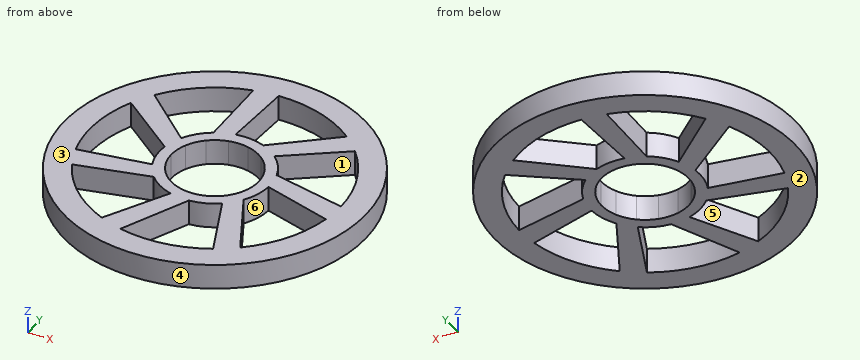
```python
from build123d import *

# Parameters (mm, degrees)
F0_R     = 38.1
F1_DEPTH = 6.35


with BuildPart() as f1:
    # F0 (on Top) → F1 (new body)
    with BuildSketch(Plane.XY):
        Circle(F0_R)
        with BuildLine():
            ThreePointArc((31.7250303997, 0), (31.5812646245, -3.0168325409), (31.1512702825, -6.0063228058))
            ThreePointArc((31.1512702825, -6.0063228058), (27.1447816525, -16.4206693804), (19.7802329179, -24.8036275488))
            ThreePointArc((19.7802329179, -24.8036275488), (17.3319417654, -26.5721912628), (14.7265670727, -28.0999248419))
            ThreePointArc((14.7265670727, -28.0999248419), (4.0862982493, -31.460764779), (-7.0594833943, -30.9296176515))
            ThreePointArc((-7.0594833943, -30.9296176515), (-9.9686867503, -30.1181479898), (-12.7875415101, -29.033710338))
            ThreePointArc((-12.7875415101, -29.033710338), (-22.049251081, -22.8102626164), (-28.5832647234, -13.7649748135))
            ThreePointArc((-28.5832647234, -13.7649748135), (-29.7626908188, -10.9845249823), (-30.6723705175, -8.1045197699))
            ThreePointArc((-30.6723705175, -8.1045197699), (-31.5812646245, 3.0168325409), (-28.5832647234, 13.7649748135))
            ThreePointArc((-28.5832647234, 13.7649748135), (-27.1447816525, 16.4206693804), (-25.4602789229, 18.9275394871))
            ThreePointArc((-25.4602789229, 18.9275394871), (-17.3319417654, 26.5721912628), (-7.0594833943, 30.9296176515))
            ThreePointArc((-7.0594833943, 30.9296176515), (-4.0862982493, 31.460764779), (-1.0760780042, 31.7067754588))
            ThreePointArc((-1.0760780042, 31.7067754588), (9.9686867503, 30.1181479898), (19.7802329179, 24.8036275488))
            ThreePointArc((19.7802329179, 24.8036275488), (22.049251081, 22.8102626164), (24.1184315996, 20.6101628097))
            ThreePointArc((24.1184315996, 20.6101628097), (29.7626908188, 10.9845249823), (31.7250303997, 0))
        make_face(mode=Mode.SUBTRACT)
        with BuildLine():
            Line((-10.2881439148, -9.4506610768), (-6.878658835, -8.6466440676))
            ThreePointArc((-6.878658835, -8.6466440676), (-8.634357457, -6.8940751595), (-9.9548050215, -4.7939814335))
            Line((-9.9548050215, -4.7939814335), (-12.9376014162, -5.270613778))
            ThreePointArc((-12.9376014162, -5.270613778), (-11.7994495804, -7.4788962822), (-10.2881439148, -9.4506610768))
        make_face()
        with BuildLine():
            Line((-28.5832647234, -13.7649748135), (-10.2881439148, -9.4506610768))
            ThreePointArc((-10.2881439148, -9.4506610768), (-11.7994495804, -7.4788962822), (-12.9376014162, -5.270613778))
            Line((-12.9376014162, -5.270613778), (-30.6723705175, -8.1045197699))
            ThreePointArc((-30.6723705175, -8.1045197699), (-29.7626908188, -10.9845249823), (-28.5832647234, -13.7649748135))
        make_face()
        with BuildLine():
            ThreePointArc((-11.0489921838, -0.0131423621), (-10.7734388222, 2.4522269355), (-9.9548050215, 4.7939814335))
            Line((-9.9548050215, 4.7939814335), (-12.187194327, 6.8288501547))
            ThreePointArc((-12.187194327, 6.8288501547), (-13.2040730485, 4.5621655966), (-13.8033771709, 2.1512040066))
            Line((-13.8033771709, 2.1512040066), (-11.0489921838, -0.0131423621))
        make_face()
        with BuildLine():
            ThreePointArc((-13.8033771709, 2.1512040066), (-13.2040730485, 4.5621655966), (-12.187194327, 6.8288501547))
            Line((-12.187194327, 6.8288501547), (-25.4602789229, 18.9275394871))
            ThreePointArc((-25.4602789229, 18.9275394871), (-27.1447816525, 16.4206693804), (-28.5832647234, 13.7649748135))
            Line((-28.5832647234, 13.7649748135), (-13.8033771709, 2.1512040066))
        make_face()
        with BuildLine():
            ThreePointArc((-6.8992090599, 8.6302558101), (-4.7999010163, 9.9519521318), (-2.4586337993, 10.7719785017))
            Line((-2.4586337993, 10.7719785017), (-2.2595813362, 13.7860506377))
            ThreePointArc((-2.2595813362, 13.7860506377), (-4.665760197, 13.16782373), (-6.9243858797, 12.1331685964))
            Line((-6.9243858797, 12.1331685964), (-6.8992090599, 8.6302558101))
        make_face()
        with BuildLine():
            ThreePointArc((-6.9243858797, 12.1331685964), (-4.665760197, 13.16782373), (-2.2595813362, 13.7860506377))
            Line((-2.2595813362, 13.7860506377), (-1.0760780042, 31.7067754588))
            ThreePointArc((-1.0760780042, 31.7067754588), (-4.0862982493, 31.460764779), (-7.0594833943, 30.9296176515))
            Line((-7.0594833943, 30.9296176515), (-6.9243858797, 12.1331685964))
        make_face()
        with BuildLine():
            ThreePointArc((2.4458192044, 10.7748953322), (4.7880601551, 9.95765439), (6.8889388207, 8.6384560498))
            Line((6.8889388207, 8.6384560498), (9.3695424879, 10.3620738064))
            ThreePointArc((9.3695424879, 10.3620738064), (7.3859652469, 11.85784202), (5.1688092106, 12.9786097616))
            Line((5.1688092106, 12.9786097616), (2.4458192044, 10.7748953322))
        make_face()
        with BuildLine():
            ThreePointArc((5.1688092106, 12.9786097616), (7.3859652469, 11.85784202), (9.3695424879, 10.3620738064))
            Line((9.3695424879, 10.3620738064), (24.1184315996, 20.6101628097))
            ThreePointArc((24.1184315996, 20.6101628097), (22.049251081, 22.8102626164), (19.7802329179, 24.8036275488))
            Line((19.7802329179, 24.8036275488), (5.1688092106, 12.9786097616))
        make_face()
        with BuildLine():
            ThreePointArc((9.9490957221, 4.8058189013), (10.770514371, 2.4650397934), (11.049, 0))
            Line((11.049, 0), (13.9432097147, -0.864755949))
            ThreePointArc((13.9432097147, -0.864755949), (13.9633008224, -0.4325854166), (13.97, 0))
            ThreePointArc((13.97, 0), (13.8191317384, 2.0475590338), (13.3697855409, 4.0508930609))
            Line((13.3697855409, 4.0508930609), (9.9490957221, 4.8058189013))
        make_face()
        with BuildLine():
            ThreePointArc((13.97, 0), (13.9633008224, -0.4325854166), (13.9432097147, -0.864755949))
            Line((13.9432097147, -0.864755949), (31.1512702825, -6.0063228058))
            ThreePointArc((31.1512702825, -6.0063228058), (31.5812646245, -3.0168325409), (31.7250303997, 0))
            Line((31.7250303997, 0), (13.3697855409, 4.0508930609))
            ThreePointArc((13.3697855409, 4.0508930609), (13.8191317384, 2.0475590338), (13.97, 0))
        make_face()
        with BuildLine():
            Line((11.5030406649, -7.9272287378), (9.9605002365, -4.7821371831))
            ThreePointArc((9.9605002365, -4.7821371831), (8.6425515871, -6.8838000453), (6.8889388207, -8.6384560498))
            Line((6.8889388207, -8.6384560498), (8.0173556368, -11.4404068369))
            ThreePointArc((8.0173556368, -11.4404068369), (9.9170092786, -9.8394017586), (11.5030406649, -7.9272287378))
        make_face()
        with BuildLine():
            Line((19.7802329179, -24.8036275488), (11.5030406649, -7.9272287378))
            ThreePointArc((11.5030406649, -7.9272287378), (9.9170092786, -9.8394017586), (8.0173556368, -11.4404068369))
            Line((8.0173556368, -11.4404068369), (14.7265670727, -28.0999248419))
            ThreePointArc((14.7265670727, -28.0999248419), (17.3319417654, -26.5721912628), (19.7802329179, -24.8036275488))
        make_face()
        with BuildLine():
            Line((0.974271549, -13.935985611), (2.4714449156, -10.7690464308))
            ThreePointArc((2.4714449156, -10.7690464308), (0.0065711822, -11.048998046), (-2.4586337993, -10.7719785017))
            Line((-2.4586337993, -10.7719785017), (-3.9457307599, -13.4011980349))
            ThreePointArc((-3.9457307599, -13.4011980349), (-1.5095999134, -13.8881967189), (0.974271549, -13.935985611))
        make_face()
        with BuildLine():
            Line((-7.0594833943, -30.9296176515), (0.974271549, -13.935985611))
            ThreePointArc((0.974271549, -13.935985611), (-1.5095999134, -13.8881967189), (-3.9457307599, -13.4011980349))
            Line((-3.9457307599, -13.4011980349), (-12.7875415101, -29.033710338))
            ThreePointArc((-12.7875415101, -29.033710338), (-9.9686867503, -30.1181479898), (-7.0594833943, -30.9296176515))
        make_face()
        with BuildLine():
            ThreePointArc((-9.9548050215, 4.7939814335), (-8.6425515871, 6.8838000453), (-6.8992090599, 8.6302558101))
            Line((-6.8992090599, 8.6302558101), (-6.9243858797, 12.1331685964))
            ThreePointArc((-6.9243858797, 12.1331685964), (-9.9170092786, 9.8394017586), (-12.187194327, 6.8288501547))
            Line((-12.187194327, 6.8288501547), (-9.9548050215, 4.7939814335))
        make_face()
        with BuildLine():
            Line((-12.9376014162, -5.270613778), (-9.9548050215, -4.7939814335))
            ThreePointArc((-9.9548050215, -4.7939814335), (-10.770514371, -2.4650397934), (-11.0489921838, -0.0131423621))
            Line((-11.0489921838, -0.0131423621), (-13.8033771709, 2.1512040066))
            ThreePointArc((-13.8033771709, 2.1512040066), (-13.8759082137, -1.6186634131), (-12.9376014162, -5.270613778))
        make_face()
        with BuildLine():
            Line((-3.9457307599, -13.4011980349), (-2.4586337993, -10.7719785017))
            ThreePointArc((-2.4586337993, -10.7719785017), (-4.7880601551, -9.95765439), (-6.878658835, -8.6466440676))
            Line((-6.878658835, -8.6466440676), (-10.2881439148, -9.4506610768))
            ThreePointArc((-10.2881439148, -9.4506610768), (-7.3859652469, -11.85784202), (-3.9457307599, -13.4011980349))
        make_face()
        with BuildLine():
            Line((8.0173556368, -11.4404068369), (6.8889388207, -8.6384560498))
            ThreePointArc((6.8889388207, -8.6384560498), (4.7999010163, -9.9519521318), (2.4714449156, -10.7690464308))
            Line((2.4714449156, -10.7690464308), (0.974271549, -13.935985611))
            ThreePointArc((0.974271549, -13.935985611), (4.665760197, -13.16782373), (8.0173556368, -11.4404068369))
        make_face()
        with BuildLine():
            Line((13.9432097147, -0.864755949), (11.049, 0))
            ThreePointArc((11.049, 0), (10.7734388222, -2.4522269355), (9.9605002365, -4.7821371831))
            Line((9.9605002365, -4.7821371831), (11.5030406649, -7.9272287378))
            ThreePointArc((11.5030406649, -7.9272287378), (13.2040730485, -4.5621655966), (13.9432097147, -0.864755949))
        make_face()
        with BuildLine():
            ThreePointArc((6.8889388207, 8.6384560498), (8.634357457, 6.8940751595), (9.9490957221, 4.8058189013))
            Line((9.9490957221, 4.8058189013), (13.3697855409, 4.0508930609))
            ThreePointArc((13.3697855409, 4.0508930609), (11.7994495804, 7.4788962822), (9.3695424879, 10.3620738064))
            Line((9.3695424879, 10.3620738064), (6.8889388207, 8.6384560498))
        make_face()
        with BuildLine():
            ThreePointArc((-2.4586337993, 10.7719785017), (-0.0065711822, 11.048998046), (2.4458192044, 10.7748953322))
            Line((2.4458192044, 10.7748953322), (5.1688092106, 12.9786097616))
            ThreePointArc((5.1688092106, 12.9786097616), (1.5095999134, 13.8881967189), (-2.2595813362, 13.7860506377))
            Line((-2.2595813362, 13.7860506377), (-2.4586337993, 10.7719785017))
        make_face()
    extrude(amount=F1_DEPTH)


solid = f1.part
```
Verification items for the finished model (mm, model axes). Face numbers are marked on the shaded views. A direction names the side the tool comes from. Coordinates: 2 decimals unless noted, no trailing zeros. Loops run counter-clockwise (first coordinate to the right, second up) from the corner with the lowest first, then second, coordinate; pieces in that order, holes last. Notation, with made-up numbers: (72, 77.5) - (79, 77.5) arc R16 cw to (79, 97.5) - close; hole circle Ø3 at (53, 11). An arc over 180 degrees is marked (long way). Answer as a JSON object with one key per item and string values.
(1) Cross-section at C-C, the plane x = -18.5. Record the boundary of the cut face in (y, z).
Response:
{"outline": "(-33.31, 0) - (-25.77, 0) - (-25.77, 6.35) - (-33.31, 6.35) - close; (-11.39, 0) - (-6.16, 0) - (-6.16, 6.35) - (-11.39, 6.35) - close; (5.84, 0) - (12.58, 0) - (12.58, 6.35) - (5.84, 6.35) - close; (25.77, 0) - (33.31, 0) - (33.31, 6.35) - (25.77, 6.35) - close"}
(2) Cross-section at D-D, the plane y = -22.5. Record the boundary of the cut face in (x, z).
Response:
{"outline": "(-30.75, 0) - (-22.37, 0) - (-22.37, 6.35) - (-30.75, 6.35) - close; (-9.09, 0) - (-3.07, 0) - (-3.07, 6.35) - (-9.09, 6.35) - close; (12.47, 0) - (18.65, 0) - (18.65, 6.35) - (12.47, 6.35) - close; (22.37, 0) - (30.75, 0) - (30.75, 6.35) - (22.37, 6.35) - close"}
(3) Go/stop test with a flat-tipped pin: pin 1 Ø2 at (x, z) = (10, 1.5) entering from -Y. Record where the tip stops, or that it passes through.
Response:
{"pin 1": "stops at y = -37.02"}
(4) Access from +Z, -Z, +X, -X, +Y, -Y to the whole of each face (thin tool, end or side, straight path). Record for the marked faces 1 and 2.
Response:
{"face 1": "+Z, -Z", "face 2": "-Z, +X, -X, +Y, -Y"}
(5) Cross-section at A-A, the plane x = 22.5. Record the boundary of the cut face in (y, z).
Response:
{"outline": "(-30.75, 0) - (-22.37, 0) - (-22.37, 6.35) - (-30.75, 6.35) - close; (-3.42, 0) - (2.04, 0) - (2.04, 6.35) - (-3.42, 6.35) - close; (19.49, 0) - (30.75, 0) - (30.75, 6.35) - (19.49, 6.35) - close"}
(6) Scan lines: line 1 along Y through (x, z) = (14, 4); line 2 along Y through (x, z) = (5, 4.75); line 3 along Y through (x, z) = (-1, 1.75). Record each from-to range of solid material in increasing order.
Response:
{"line 1": "y = -35.43 to -28.47, -26.3 to -13.02, -0.88 to 3.91, 13.58 to 20.13, 28.47 to 35.43", "line 2": "y = -37.77 to -31.33, -13.04 to -9.85, 9.85 to 13.04, 31.33 to 37.77", "line 3": "y = -38.09 to -31.71, -18.11 to -11, 11 to 13.93, 31.71 to 38.09"}
(7) Cross-section at B-B, the plane y = 27. Record the boundary of the cut face in (x, z).
Response:
{"outline": "(-26.88, 0) - (-16.66, 0) - (-16.66, 6.35) - (-26.88, 6.35) - close; (-7.03, 0) - (-1.39, 0) - (-1.39, 6.35) - (-7.03, 6.35) - close; (16.66, 0) - (26.88, 0) - (26.88, 6.35) - (16.66, 6.35) - close"}
(8) Mould release check, pull along Y, two halves, no side actions. Record for the marked faces 3, 4, 5 and 6: pulls with the +Y half, pulls with the -Y half, needs draft (parallel to the pull), parting line crosses it, or undercut.
Response:
{"face 3": "needs draft", "face 4": "parting line crosses it", "face 5": "undercut", "face 6": "undercut"}
